Check sheet for the modelled part. Datum: model origin and axes. Units: mm. A direction names the side the tool comes from. Coordinates: 2 decimals unless noted, no trailing zeros. Write each loop counter-clockwise with the first axis right and the second up, starting at its lowest first coordinate (ties: lowest second). Pieces come first, ordered by that corner, then holes. Notation, with made-up numbers: (-39.5, 27) -> (0.5, 27) arc R9 ccw to (0.5, 36) -> close; hole circle Ø10 at (22.25, 39.5). An arc over 180 degrees is marked (long way). One line per item, written item: value. Start each with the question number.
1) Set-up check for faces 1 (the cylindrical face through (45, 3, -75)), 2 (the flat face through (100, 2, -1)), 3 (the flat face through (-20, 2, -23)): record each of +Z, -Z, +X, -X, +Y, -Y from which the full face is reachable in a straight line by a thin tool's end or side.
2) Draft check along X on faces 4 (the flat face through (23, 2, -24)), 5 (the flat face through (1, 0, 1)), 6 (the flat face through (-100, 2, 1)). Enter one of: +X half, -X half, draft (parallel to the pull), parting line (faces both ways), or undercut.
3) Gauge pin test, flat ends, axial feed: P1, Ø3, axis at x = 20.5, z = 21, coming from the -Y side; P2, Ø4.5, axis at x = -22, z = -22, coming from the -Y side; P3, Ø3.5, axis at x = 22, z = -22, coming from the +Y side. Record the tip position at first contact, or that the pin passes through.
4) Scan lines: line 1 along Z through (x, y) = (32, 1.7); line 2 along Z through (x, y) = (-22, 4.25); line 3 along Z through (x, y) = (-22, 1.35). Record each from-to range of solid material in increasing order. Write a range as [from, to].
5) Sectioned sample at A-A on y = 3.85. Enter the section's corners in (x, z), plus the area to 3 significant figures.
6) Sectioned sample at C-C on z = 81.5. Enter the section's corners in (x, y).
7) Sectioned sample at B-B on z = -75. Enter the section's corners in (x, y).
Autodesk Inventor part; units mm, degrees
ref_plane "YZ Plane" through (0, 0, 0) normal (1, 0, 0) x (0, 1, 0)
ref_plane "XZ Plane" through (0, 0, 0) normal (0, 1, 0) x (-1, 0, 0)
ref_plane "XY Plane" through (0, 0, 0) normal (0, 0, 1) x (1, 0, 0)
sketch "Sketch1" plane through (0, 0, 0) normal (0, 1, 0) x (-1, 0, 0)
  line L0 (-100, 100) -> (100, 100)
  line L1 (100, 100) -> (100, -100)
  line L2 (100, -100) -> (-100, -100)
  line L3 (-100, -100) -> (-100, 100)
  line L4 (-100, 100) -> (100, -100) construction
  line L5 (100, 100) -> (-100, -100) construction
  point P0 (0, 0)
  dimension "d0" = 200
  dimension "d1" = 200
extrude "Extrusion1" add sketch "Sketch1" along normal blind 5
sketch "Sketch6" plane through (0, 0, 0) normal (0, -1, 0) x (1, 0, 0)
  line L0 (-22, 22) -> (22, 22)
  line L1 (22, 22) -> (22, -22)
  line L2 (22, -22) -> (-22, -22)
  line L3 (-22, -22) -> (-22, 22)
  line L4 (-22, 22) -> (22, -22) construction
  line L5 (22, 22) -> (-22, -22) construction
  point P0 (0, 0)
  dimension "d10" = 44
  dimension "d11" = 44
hole "Hole1" at (22, 0, 22) at (22, 0, -22) at (-22, 0, -22) at (-22, 0, 22) direction (0, 1, 0) diameter 4 depth 49.3
sketch "Sketch7" plane through (0, 0, 0) normal (0, -1, 0) x (1, 0, 0)
  circle A0 centre (-22, 22) radius 2
  circle A1 centre (-22, 22) radius 3
  circle A2 centre (22, 22) radius 2
  circle A3 centre (22, 22) radius 3
  circle A4 centre (-22, -22) radius 2
  circle A5 centre (-22, -22) radius 3
  circle A6 centre (22, -22) radius 3
  point P0 (0, 0)
  dimension "d19" = 6
  dimension "d20" = 6
  dimension "d21" = 6
  dimension "d22" = 6
extrude "Extrusion3" cut sketch "Sketch7" against normal blind 2 contours A0 | A1 | A3 | A5 | A6
sketch "Sketch13" plane through (0, 5, 0) normal (0, 1, 0) x (1, 0, 0)
  line L0 (-35, 75) -> (35, 75) construction
  line L1 (-35, 65) -> (35, 65)
  line L2 (35, 85) -> (-35, 85)
  arc A0 (-35, 85) -> (-35, 65) centre (-35, 75) ccw
  arc A1 (35, 65) -> (35, 85) centre (35, 75) ccw
  line L3 (-35, 75) -> (-35, -100)
  line L4 (-100, -100) -> (100, -100)
  line L5 (35, 75) -> (35, -100)
  line L6 (-35, -75) -> (35, -75) construction
  line L7 (-35, -85) -> (35, -85)
  line L8 (35, -65) -> (-35, -65)
  arc A2 (-35, -65) -> (-35, -85) centre (-35, -75) ccw
  arc A3 (35, -85) -> (35, -65) centre (35, -75) ccw
  line L9 (-50, 50) -> (50, 50)
  line L10 (50, 50) -> (50, -50)
  line L11 (50, -50) -> (-50, -50)
  line L12 (-50, -50) -> (-50, 50)
  line L13 (-50, 50) -> (50, -50) construction
  line L14 (50, 50) -> (-50, -50) construction
  line L15 (16.6148, -50) -> (16.6148, -65)
  line L16 (16.6148, -85) -> (16.6148, -100)
  line L17 (31.6927, 50) -> (31.6927, 65)
  point P0 (0, 0)
  point P1 (-100, 100)
  point P2 (0, 75)
  point P3 (0, -75)
  dimension "d56" = 20
  dimension "d59" = 20
  dimension "d60" = 100
  dimension "d61" = 100
  dimension "d62" = 15
  dimension "d64" = 15
extrude "Extrusion5" cut sketch "Sketch13" against normal blind 5 contours A0 L2 A1 L1 | L8 L5 L7 L3 | L3 A2 | A3 L5
sketch "Sketch14" plane through (0, 5, 0) normal (0, 1, 0) x (1, 0, 0)
  point P0 (0, 0)
properties part number "Base myCobot_3DPrint"
Answers:
1. face 1: +Y, -Y
1. face 2: +Z, -Z, +X, +Y, -Y
1. face 3: -Y
2. face 4: undercut
2. face 5: draft
2. face 6: -X half
3. P1: stops at y = 0
3. P2: stops at y = 2
3. P3: passes through
4. line 1: z = [-100, -85], [-65, 65], [85, 100]
4. line 2: z = [-100, -85], [-65, -24], [-20, 20], [24, 65], [85, 100]
4. line 3: z = [-100, -85], [-65, -25], [-19, 19], [25, 65], [85, 100]
5. outline: (-100, -100) -> (100, -100) -> (100, 100) -> (-100, 100) -> close; hole (-35, -85) -> (35, -85) arc R10 ccw to (35, -65) -> (-35, -65) arc R10 ccw to start; hole (-35, 65) -> (35, 65) arc R10 ccw to (35, 85) -> (-35, 85) arc R10 ccw to start; hole circle Ø4 at (-22, -22); hole circle Ø4 at (-22, 22); hole circle Ø4 at (22, -22); hole circle Ø4 at (22, 22)
5. area: 36,500 mm2
6. outline: (-100, 0) -> (-42.6, 0) -> (-42.6, 5) -> (-100, 5) -> close; (42.6, 0) -> (100, 0) -> (100, 5) -> (42.6, 5) -> close
7. outline: (-100, 0) -> (-45, 0) -> (-45, 5) -> (-100, 5) -> close; (45, 0) -> (100, 0) -> (100, 5) -> (45, 5) -> close
